from build123d import *

# Parameters (mm, degrees)
SKETCH_1_W               = 50
SKETCH_1_H               = 40
EXTRUDE_1_DEPTH          = 4
SKETCH_2_R               = 12.5
EXTRUDE_2_DEPTH          = 25
SKETCH_3_W               = 10
SKETCH_3_H               = 20
CUT_EXTRUDE_1_DEPTH      = 20
SKETCH_4_R               = 4
CUT_EXTRUDE_2_DEPTH      = 26
CUT_EXTRUDE_2_DEPTH_BACK = 26
SKETCH_5_R               = 2.5
CUT_EXTRUDE_3_DEPTH      = 10


with BuildPart() as part:
    # 草图1 → 凸台-拉伸1 (new body)
    with BuildSketch(Plane(origin=(0, 0, 0), x_dir=(1, 0, 0), z_dir=(0, 1, 0))):
        Rectangle(SKETCH_1_W, SKETCH_1_H)
    extrude(amount=EXTRUDE_1_DEPTH)

    # 草图2 → 凸台-拉伸2 (add)
    with BuildSketch(Plane(origin=(0, 4, 0), x_dir=(1, 0, 0), z_dir=(0, 1, 0))):
        Circle(SKETCH_2_R)
    extrude(amount=EXTRUDE_2_DEPTH)

    # 草图3 → 切除-拉伸1 (cut, symmetric)
    with BuildSketch(Plane.XY):
        with Locations((0, 19)):
            Rectangle(SKETCH_3_W, SKETCH_3_H)
    extrude(amount=CUT_EXTRUDE_1_DEPTH, both=True, mode=Mode.SUBTRACT)

    # 草图4 → 切除-拉伸2 (cut, two sides)
    with BuildSketch(Plane(origin=(0, 0, 0), x_dir=(0, 0, -1), z_dir=(1, 0, 0))) as cut_extrude_2_sk:
        with Locations((0, 19)):
            Circle(SKETCH_4_R)
    extrude(amount=CUT_EXTRUDE_2_DEPTH, mode=Mode.SUBTRACT)
    extrude(cut_extrude_2_sk.sketch, amount=-CUT_EXTRUDE_2_DEPTH_BACK, mode=Mode.SUBTRACT)

    # 草图5 → 切除-拉伸3 (cut)
    with BuildSketch(Plane(origin=(0, 4, 0), x_dir=(1, 0, 0), z_dir=(0, 1, 0))):
        with Locations((-21, 0)):
            Circle(SKETCH_5_R)
        with Locations((21, 0)):
            Circle(SKETCH_5_R)
    extrude(amount=-CUT_EXTRUDE_3_DEPTH, mode=Mode.SUBTRACT)


solid = part.part
Can you work these out from the model? Positions are in its coordinate system, mm. A direction names the side the tool comes from. Round coordinates to 2 decimals unless told otherwise and drop trailing zeros. Loops run counter-clockwise (first coordinate to the right, second up) from the corner with the lowest first, then second, coordinate; pieces in that order, holes last. Notation, with made-up numbers: (79.5, -9.75) - (120.5, -9.75) arc R37 ccw to (120.5, 26.25) - close; hole circle Ø11 at (17.25, -33). An arc over 180 degrees is marked (long way). Write item = value, one per line. Start each with the question number.
(1) If I drill on probe 1 along X at (y, z) = (1.7, 0); probe 2 along Z at (x, y) = (21, 3.15); probe 3 along Y at (x, z) = (7.75, 0), over which ranges is the centre line in solid material (lowest first)? Write a range as [from, to].
(2) If we section it at D-D (x = 0): Please give me the cut outline in (y, z), and give its area (3 significant figures).
(3) If we section it at A-A (x = 21): Please give me the cut outline in (y, z).
(4) If we section it at C-C (y = 26.5): Please give me the cut outline in (x, z).
(5) For P1, Ø3, axis at y = 13.5, z = -1.5, coming from the +X side; P2, Ø5, axis at x = -3, y = 11, coming from the +Z side; P3, Ø4, axis at y = 8, z = 2.5, coming from the -X side; P4, Ø4, axis at x = 21, z = 0, coming from the -Y side, each with a flat end and sliding along its axis, tell me the tip position at first contact or that it passes through.
(6) For faces 1 (the face through (0, 9, 0)), 2 (the face through (25, 2, 0)), 3 (the face through (0, 4, -14)), which set-ups out of +Z, -Z, +X, -X, +Y, -Y let a thin tool reach every point of the face, with its end or its side?
(7) If we mould it in two halves opening along X, with no side actions, what happens to faces 4 (the face through (11.547, 16.325, 4.788)), 5 (the face through (-5, 14, 0)), 6 (the face through (8, 29, 0))? For each: released by +X, released by -X, zero draft, split by the parting line, or undercut.
(8) If we section it at B-B (z = 0): Please give me the cut outline in (x, y), and give its area (3 significant figures).
Ans:
q1.probe_1 = [-25, -23.5], [-18.5, 18.5], [23.5, 25]
q1.probe_2 = [-20, -2.5], [2.5, 20]
q1.probe_3 = [0, 15], [23, 29]
q2.outline = (0, -20) - (4, -20) - (4, -12.5) - (9, -12.5) - (9, 12.5) - (4, 12.5) - (4, 20) - (0, 20) - close
q2.area = 285 mm²
q3.outline = (0, -20) - (4, -20) - (4, -2.5) - (0, -2.5) - close; (0, 2.5) - (4, 2.5) - (4, 20) - (0, 20) - close
q4.outline = (-5, -11.46) - (-5, 11.46) arc R12.5 ccw to start; (5, -11.46) arc R12.5 ccw to (5, 11.46) - close
q5.P1 = 12.5
q5.P2 = 12.41
q5.P3 = -12.49
q5.P4 = through
q6.face_1 = +Z, -Z, +Y
q6.face_2 = +Z, -Z, +X, +Y, -Y
q6.face_3 = +Y
q7.face_4 = split by the parting line
q7.face_5 = undercut
q7.face_6 = zero draft
q8.outline = (-25, 0) - (-23.5, 0) - (-23.5, 4) - (-25, 4) - close; (-18.5, 0) - (18.5, 0) - (18.5, 4) - (12.5, 4) - (12.5, 15) - (5, 15) - (5, 9) - (-5, 9) - (-5, 15) - (-12.5, 15) - (-12.5, 4) - (-18.5, 4) - close; (-12.5, 23) - (-5, 23) - (-5, 29) - (-12.5, 29) - close; (5, 23) - (12.5, 23) - (12.5, 29) - (5, 29) - close; (23.5, 0) - (25, 0) - (25, 4) - (23.5, 4) - close
q8.area = 465 mm²
